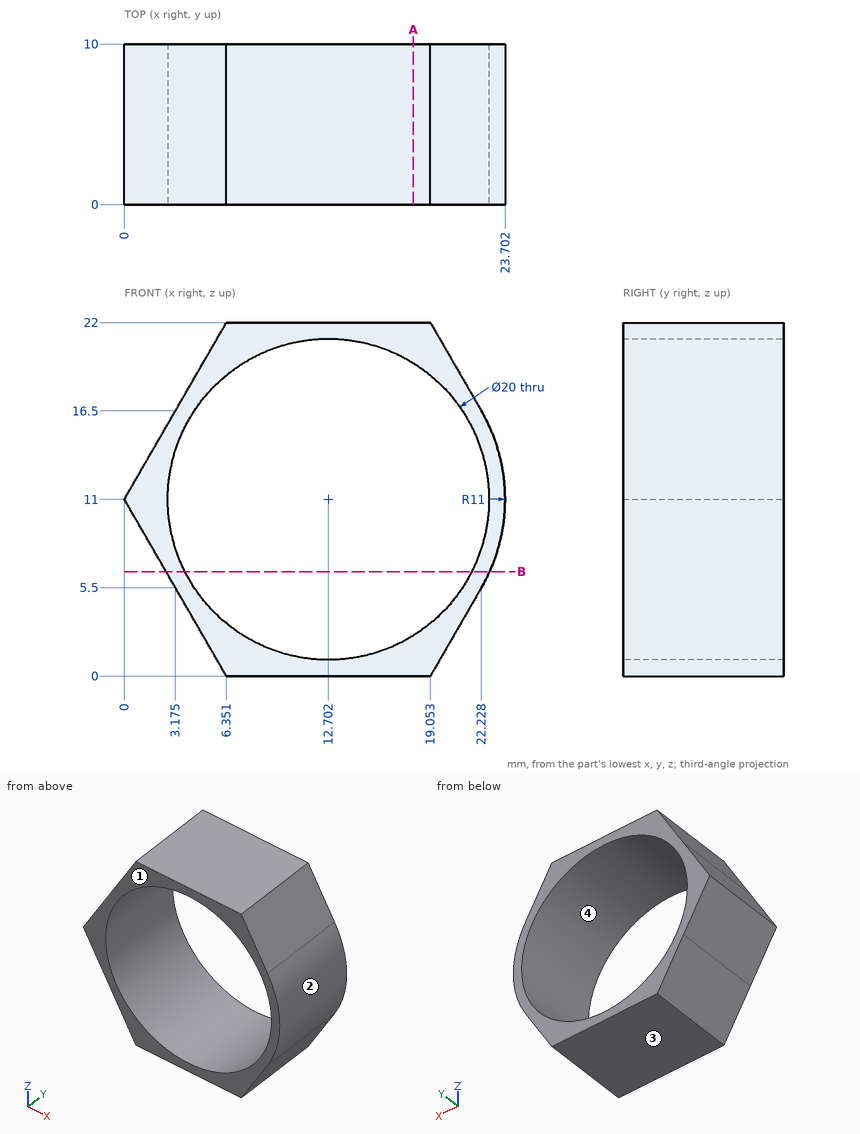
Here's the drawing with two shaded views (mm, measured from the low corner). I have some questions. Coordinates: 2 decimals unless noted, no trailing zeros. Write each loop counter-clockwise with the first axis right and the second up, starting at its lowest first coordinate (ties: lowest second). Pieces come first, ordered by that corner, then holes. Notation, with made-up numbers: (15.5, 65.25) -> (38.5, 65.25) arc R20 ccw to (38.5, 91.25) -> close; hole circle Ø5 at (18, 60). An arc over 180 degrees is marked (long way). Write item = value, one per line. Start each with the question number.
(1) Will this pin go through, and if not, where does the flat tip stop? pin 1 (5 mm diameter, centred on x = 18.5, z = 7, fed in from +Y).
(2) I want a section at B-B (z = 6.5). Please give me the cut outline in (x, y), plus the area to 3 significant figures.
(3) I want a section at A-A (x = 18). Please give me the cut outline in (y, z).
(4) We'd pull the mould along Z, two halves only. Please class the marked faces 1, 2, 3 and 4: released by +Z, released by -Z, zero draft, split by the parting line, or undercut.
(5) I need wall thicknesses on line 1 (Z direction, x = 12.25, y = 9.5); line 2 (Z direction, x = 6.5, y = 0.75) (1 decimal); line 3 (X direction, y = 2.5, z = 9.5) (1 decimal). Which ranges of each line are inside material? Lowest first, please. Write a range as [from, to].
Result set:
q1.pin_1 = through
q2.outline = (2.6, 0) -> (3.77, 0) -> (3.77, 10) -> (2.6, 10) -> close; (21.63, 0) -> (22.74, 0) -> (22.74, 10) -> (21.63, 10) -> close
q2.area = 22.8 mm2
q3.outline = (0, 0) -> (10, 0) -> (10, 2.52) -> (0, 2.52) -> close; (0, 19.48) -> (10, 19.48) -> (10, 22) -> (0, 22) -> close
q4.face_1 = zero draft
q4.face_2 = split by the parting line
q4.face_3 = released by -Z
q4.face_4 = undercut
q5.line_1 = [0, 1.01], [20.99, 22]
q5.line_2 = [0, 3.2], [18.8, 22]
q5.line_3 = [0.9, 2.8], [22.6, 23.6]
